Check sheet for the modelled part. Datum: model origin and axes. Units: mm. A direction names the side the tool comes from. Give positions to 0.01 mm unless a question says otherwise; leave off trailing zeros. Loops run counter-clockwise (first coordinate to the right, second up) from the corner with the lowest first, then second, coordinate; pieces in that order, holes last. Notation, with made-up numbers: (58, 26.25) - (114, 26.25) arc R27 ccw to (114, 59.25) - close; hole circle Ø1 at (80, 60). An arc over 180 degrees is marked (long way). Answer in a Markdown table with one row per item. Add a question column.
(1) Thickness scan on L1, parallel to X at y = 1.5, z = 0; L2, parallel to X at y = 4.5, z = 6.25; L3, parallel to Y at x = 3.5, z = -2. Record the ranges inside material, lowest first.
(2) Sectioned sample at D-D on z = -3. Enter the section's corners in (x, y).
(3) Draft check along Z on faces 1 (the face through (8.259, 2.251, -3.307)), 2 (the face through (0.1, 1.8, -6.5)), 3 (the face through (9.5, 4.2, 0.1)), 4 (the face through (-8, 4, 0)). Enter one of: released by +Z, released by -Z, zero draft, split by the parting line, or undercut.
(4) Sectioned sample at A-A on x = 0. Enter the section's corners in (y, z), then the cut area to 3 significant figures.
(5) Go/stop test with flat-tipped pins: P1, Ø5, axis at x = 0, z = 0, coming from the +Y side; P2, Ø3, axis at x = -3, y = 5, coming from the +Z side. Record where each tip stops, or that it passes through.
(6) Sectioned sample at B-B on z = 0. Enter the section's corners in (x, y), then the cut area to 3 significant figures.
(7) Set-up check for faces 5 (the face through (7, 5, 0)), 6 (the face through (8.26, 2.24, 3.3)), 7 (the face through (-2.1, 0, -1.4)): record each of +Z, -Z, +X, -X, +Y, -Y from which the full face is reachable in a straight line by a thin tool's end or side.
(8) Sectioned sample at C-C on y = 4.25. Enter the section's corners in (x, z).
from build123d import *

# Parameters (mm, degrees)
SKETCH1_W               = 19
SKETCH1_H               = 13
SKETCH1_R               = 2.159
BOSS_EXTRUDE1_DEPTH     = 2
BOSS_EXTRUDE2_DEPTH     = 19
CUT_EXTRUDE1_DEPTH      = 18.363755354
CUT_EXTRUDE1_DEPTH_BACK = 18.363755354
SKETCH4_W               = 14
SKETCH4_H               = 5
FILLET1_R               = 0.75
CHAMFER1_SIZE           = 0.5


with BuildPart() as part:
    # Sketch1 → Boss-Extrude1 (new body)
    with BuildSketch(Plane(origin=(0, 0, 0), x_dir=(1, 0, 0), z_dir=(0, 1, 0))):
        Rectangle(SKETCH1_W, SKETCH1_H)
        with Locations(Location((0, 0, 0), (0, 0, 270))):
            Circle(SKETCH1_R, mode=Mode.SUBTRACT)
    extrude(amount=BOSS_EXTRUDE1_DEPTH)

    # Sketch2 → Boss-Extrude2 (add)
    with BuildSketch(Plane(origin=(9.5, 0, 0), x_dir=(0, 0, -1), z_dir=(1, 0, 0))):
        with BuildLine():
            Line((-6.5, 5.2), (-6.5, 2))
            Line((-6.5, 2), (-3.5, 2))
            Line((-3.5, 2), (-3.5, 2.7))
            ThreePointArc((-3.5, 2.7), (-3.119238816, 3.619238816), (-2.2, 4))
            Line((-2.2, 4), (2.2, 4))
            ThreePointArc((2.2, 4), (3.119238816, 3.619238816), (3.5, 2.7))
            Line((3.5, 2.7), (3.5, 2))
            Line((3.5, 2), (6.5, 2))
            Line((6.5, 2), (6.5, 5.2))
            ThreePointArc((6.5, 5.2), (6.119238816, 6.119238816), (5.2, 6.5))
            Line((5.2, 6.5), (-5.2, 6.5))
            ThreePointArc((-5.2, 6.5), (-6.119238816, 6.119238816), (-6.5, 5.2))
        make_face()
    extrude(amount=-BOSS_EXTRUDE2_DEPTH)

    # Sketch4 → Cut-Extrude1 (cut, two sides: drawn at the far end of the back side and taken through both)
    with BuildSketch(Plane.XY.offset(6.5).offset(-CUT_EXTRUDE1_DEPTH_BACK)):
        with Locations((0, 4.5)):
            Rectangle(SKETCH4_W, SKETCH4_H)
    extrude(amount=CUT_EXTRUDE1_DEPTH + CUT_EXTRUDE1_DEPTH_BACK, mode=Mode.SUBTRACT)

    # Fillet1
    # the kernel refuses this fillet: 0.75 mm, written as the material it adds along each edge
    with BuildSketch(Plane(origin=(-7, 2, 3.5), x_dir=(1, 0, 0), z_dir=(0, 0, 1)), Plane(origin=(-7, 2, -6.5), x_dir=(1, 0, 0), z_dir=(0, 0, 1))) as fillet1_piece_1:
        with BuildLine():
            CenterArc((FILLET1_R, FILLET1_R), FILLET1_R, 180, 90)
            Line((0, FILLET1_R), (-FILLET1_R * 0.02, FILLET1_R))
            Line((-FILLET1_R * 0.02, FILLET1_R), (-FILLET1_R * 0.02, -FILLET1_R * 0.02))
            Line((-FILLET1_R * 0.02, -FILLET1_R * 0.02), (FILLET1_R, -FILLET1_R * 0.02))
            Line((FILLET1_R, -FILLET1_R * 0.02), (FILLET1_R, 0))
        make_face()
    extrude(amount=3)
    with BuildSketch(Plane(origin=(-7, 2, 3.5), x_dir=(0, 0, -1), z_dir=(-1, 0, 0)), Plane(origin=(9.5, 2, 3.5), x_dir=(0, 0, -1), z_dir=(-1, 0, 0))) as fillet1_piece_2:
        with BuildLine():
            CenterArc((0.752277442, -0.75), FILLET1_R, 90, 95.21590857)
            Line((0.005383046, -0.818181818), (-0.069306394, -0.825))
            ThreePointArc((-0.069306394, -0.825), (-0.075, -0.7), (-0.075, 0))
            Line((-0.075, 0), (0, 0.075))
            Line((0, 0.075), (0.752277442, 0.075))
            Line((0.752277442, 0.075), (0.752277442, 0))
        make_face()
    extrude(amount=2.5)
    with BuildSketch(Plane(origin=(7, 2, 6.5), x_dir=(0, 1, 0), z_dir=(0, 0, -1)), Plane(origin=(7, 2, -3.5), x_dir=(0, 1, 0), z_dir=(0, 0, -1))) as fillet1_piece_3:
        with BuildLine():
            CenterArc((FILLET1_R, -FILLET1_R), FILLET1_R, 90, 90)
            Line((0, -FILLET1_R), (-FILLET1_R * 0.02, -FILLET1_R))
            Line((-FILLET1_R * 0.02, -FILLET1_R), (-FILLET1_R * 0.02, FILLET1_R * 0.02))
            Line((-FILLET1_R * 0.02, FILLET1_R * 0.02), (FILLET1_R, FILLET1_R * 0.02))
            Line((FILLET1_R, FILLET1_R * 0.02), (FILLET1_R, 0))
        make_face()
    extrude(amount=3)
    with BuildSketch(Plane(origin=(9.5, 2, -3.5), x_dir=(0, 0, 1), z_dir=(-1, 0, 0)), Plane(origin=(-7, 2, -3.5), x_dir=(0, 0, 1), z_dir=(-1, 0, 0))) as fillet1_piece_4:
        with BuildLine():
            CenterArc((0.752277442, 0.75), FILLET1_R, 174.78409143, 95.21590857)
            Line((0.005383046, 0.818181818), (-0.069306394, 0.825))
            ThreePointArc((-0.069306394, 0.825), (-0.075, 0.7), (-0.075, 0))
            Line((-0.075, 0), (0, -0.075))
            Line((0, -0.075), (0.752277442, -0.075))
            Line((0.752277442, -0.075), (0.752277442, 0))
        make_face()
    extrude(amount=2.5)
    with BuildSketch(Plane(origin=(-7, 2, 1.625), x_dir=(1, 0, 0), z_dir=(0, 0, 1))) as fillet1_piece_5a_section:
        with BuildLine():
            CenterArc((FILLET1_R, FILLET1_R), FILLET1_R, 180, 90)
            Line((0, FILLET1_R), (-FILLET1_R * 0.02, FILLET1_R))
            Line((-FILLET1_R * 0.02, FILLET1_R), (-FILLET1_R * 0.02, -FILLET1_R * 0.02))
            Line((-FILLET1_R * 0.02, -FILLET1_R * 0.02), (FILLET1_R, -FILLET1_R * 0.02))
            Line((FILLET1_R, -FILLET1_R * 0.02), (FILLET1_R, 0))
        make_face()
    fillet1_piece_5a = extrude(amount=4.875, mode=Mode.PRIVATE)
    fillet1_piece_5a = split(fillet1_piece_5a, bisect_by=Plane(origin=(-6.830203664, 2.169796336, 3.5), z_dir=(0, 0, -1)), keep=Keep.TOP, mode=Mode.PRIVATE)
    with BuildSketch(Plane(origin=(-4.954501184, 2, 3.5), x_dir=(0, 0, -1), z_dir=(-1, 0, 0))) as fillet1_piece_5b_section:
        with BuildLine():
            CenterArc((0.752277442, -0.75), FILLET1_R, 90, 95.21590857)
            Line((0.005383046, -0.818181818), (-0.069306394, -0.825))
            ThreePointArc((-0.069306394, -0.825), (-0.075, -0.7), (-0.075, 0))
            Line((-0.075, 0), (0, 0.075))
            Line((0, 0.075), (0.752277442, 0.075))
            Line((0.752277442, 0.075), (0.752277442, 0))
        make_face()
    fillet1_piece_5b = extrude(amount=4.545498816, mode=Mode.PRIVATE)
    fillet1_piece_5b = split(fillet1_piece_5b, bisect_by=Plane(origin=(-7, 2.182819777, 3.341220423), z_dir=(1, 0, 0)), keep=Keep.TOP, mode=Mode.PRIVATE)
    fillet1_piece_5 = fillet1_piece_5a & fillet1_piece_5b
    add(fillet1_piece_5)
    with BuildSketch(Plane(origin=(7, 2, 6.5), x_dir=(0, 1, 0), z_dir=(0, 0, -1))) as fillet1_piece_6a_section:
        with BuildLine():
            CenterArc((FILLET1_R, -FILLET1_R), FILLET1_R, 90, 90)
            Line((0, -FILLET1_R), (-FILLET1_R * 0.02, -FILLET1_R))
            Line((-FILLET1_R * 0.02, -FILLET1_R), (-FILLET1_R * 0.02, FILLET1_R * 0.02))
            Line((-FILLET1_R * 0.02, FILLET1_R * 0.02), (FILLET1_R, FILLET1_R * 0.02))
            Line((FILLET1_R, FILLET1_R * 0.02), (FILLET1_R, 0))
        make_face()
    fillet1_piece_6a = extrude(amount=4.875, mode=Mode.PRIVATE)
    fillet1_piece_6a = split(fillet1_piece_6a, bisect_by=Plane(origin=(6.830203664, 2.169796336, 3.5), z_dir=(0, 0, -1)), keep=Keep.TOP, mode=Mode.PRIVATE)
    with BuildSketch(Plane(origin=(9.5, 2, 3.5), x_dir=(0, 0, -1), z_dir=(-1, 0, 0))) as fillet1_piece_6b_section:
        with BuildLine():
            CenterArc((0.752277442, -0.75), FILLET1_R, 90, 95.21590857)
            Line((0.005383046, -0.818181818), (-0.069306394, -0.825))
            ThreePointArc((-0.069306394, -0.825), (-0.075, -0.7), (-0.075, 0))
            Line((-0.075, 0), (0, 0.075))
            Line((0, 0.075), (0.752277442, 0.075))
            Line((0.752277442, 0.075), (0.752277442, 0))
        make_face()
    fillet1_piece_6b = extrude(amount=4.545498816, mode=Mode.PRIVATE)
    fillet1_piece_6b = split(fillet1_piece_6b, bisect_by=Plane(origin=(7, 2.182819777, 3.341220423), z_dir=(-1, 0, 0)), keep=Keep.TOP, mode=Mode.PRIVATE)
    fillet1_piece_6 = fillet1_piece_6a & fillet1_piece_6b
    add(fillet1_piece_6)
    with BuildSketch(Plane(origin=(7, 2, -1.625), x_dir=(0, 1, 0), z_dir=(0, 0, -1))) as fillet1_piece_7a_section:
        with BuildLine():
            CenterArc((FILLET1_R, -FILLET1_R), FILLET1_R, 90, 90)
            Line((0, -FILLET1_R), (-FILLET1_R * 0.02, -FILLET1_R))
            Line((-FILLET1_R * 0.02, -FILLET1_R), (-FILLET1_R * 0.02, FILLET1_R * 0.02))
            Line((-FILLET1_R * 0.02, FILLET1_R * 0.02), (FILLET1_R, FILLET1_R * 0.02))
            Line((FILLET1_R, FILLET1_R * 0.02), (FILLET1_R, 0))
        make_face()
    fillet1_piece_7a = extrude(amount=4.875, mode=Mode.PRIVATE)
    fillet1_piece_7a = split(fillet1_piece_7a, bisect_by=Plane(origin=(6.830203664, 2.169796336, -3.5), z_dir=(0, 0, 1)), keep=Keep.TOP, mode=Mode.PRIVATE)
    with BuildSketch(Plane(origin=(9.5, 2, -3.5), x_dir=(0, 0, 1), z_dir=(-1, 0, 0))) as fillet1_piece_7b_section:
        with BuildLine():
            CenterArc((0.752277442, 0.75), FILLET1_R, 174.78409143, 95.21590857)
            Line((0.005383046, 0.818181818), (-0.069306394, 0.825))
            ThreePointArc((-0.069306394, 0.825), (-0.075, 0.7), (-0.075, 0))
            Line((-0.075, 0), (0, -0.075))
            Line((0, -0.075), (0.752277442, -0.075))
            Line((0.752277442, -0.075), (0.752277442, 0))
        make_face()
    fillet1_piece_7b = extrude(amount=4.545498816, mode=Mode.PRIVATE)
    fillet1_piece_7b = split(fillet1_piece_7b, bisect_by=Plane(origin=(7, 2.182819777, -3.341220423), z_dir=(-1, 0, 0)), keep=Keep.TOP, mode=Mode.PRIVATE)
    fillet1_piece_7 = fillet1_piece_7a & fillet1_piece_7b
    add(fillet1_piece_7)
    with BuildSketch(Plane(origin=(-4.954501184, 2, -3.5), x_dir=(0, 0, 1), z_dir=(-1, 0, 0))) as fillet1_piece_8a_section:
        with BuildLine():
            CenterArc((0.752277442, 0.75), FILLET1_R, 174.78409143, 95.21590857)
            Line((0.005383046, 0.818181818), (-0.069306394, 0.825))
            ThreePointArc((-0.069306394, 0.825), (-0.075, 0.7), (-0.075, 0))
            Line((-0.075, 0), (0, -0.075))
            Line((0, -0.075), (0.752277442, -0.075))
            Line((0.752277442, -0.075), (0.752277442, 0))
        make_face()
    fillet1_piece_8a = extrude(amount=4.545498816, mode=Mode.PRIVATE)
    fillet1_piece_8a = split(fillet1_piece_8a, bisect_by=Plane(origin=(-7, 2.182819777, -3.341220423), z_dir=(1, 0, 0)), keep=Keep.TOP, mode=Mode.PRIVATE)
    with BuildSketch(Plane(origin=(-7, 2, -6.5), x_dir=(1, 0, 0), z_dir=(0, 0, 1))) as fillet1_piece_8b_section:
        with BuildLine():
            CenterArc((FILLET1_R, FILLET1_R), FILLET1_R, 180, 90)
            Line((0, FILLET1_R), (-FILLET1_R * 0.02, FILLET1_R))
            Line((-FILLET1_R * 0.02, FILLET1_R), (-FILLET1_R * 0.02, -FILLET1_R * 0.02))
            Line((-FILLET1_R * 0.02, -FILLET1_R * 0.02), (FILLET1_R, -FILLET1_R * 0.02))
            Line((FILLET1_R, -FILLET1_R * 0.02), (FILLET1_R, 0))
        make_face()
    fillet1_piece_8b = extrude(amount=4.875, mode=Mode.PRIVATE)
    fillet1_piece_8b = split(fillet1_piece_8b, bisect_by=Plane(origin=(-6.830203664, 2.169796336, -3.5), z_dir=(0, 0, 1)), keep=Keep.TOP, mode=Mode.PRIVATE)
    fillet1_piece_8 = fillet1_piece_8a & fillet1_piece_8b
    add(fillet1_piece_8)

    # Chamfer1
    chamfer1_edges = [part.edges().sort_by_distance(p)[0] for p in [
        (0, 0, 6.5),
        (-9.5, 0, 0),
        (0, 0, -6.5),
        (9.5, 0, 0),
    ]]
    chamfer(chamfer1_edges, length=CHAMFER1_SIZE)


solid = part.part
Reply:
| question | item | result |
|---|---|---|
| 1 | L1 | -9.5 to -2.16, 2.16 to 9.5 |
| 1 | L2 | -9.5 to -7, 7 to 9.5 |
| 1 | L3 | 0 to 2 |
| 2 | outline | (-9.5, 0.5) - (-9, 0) - (9, 0) - (9.5, 0.5) - (9.5, 2.04) - (6.5, 2.04) arc R0.75 cw to (6.25, 2) - (-6.25, 2) arc R0.75 cw to (-6.5, 2.04) - (-9.5, 2.04) - close; (-9.5, 3.72) - (-7, 3.72) - (-7, 6.5) - (-9.5, 6.5) - close; (7, 3.72) - (9.5, 3.72) - (9.5, 6.5) - (7, 6.5) - close |
| 3 | face 1 | undercut |
| 3 | face 2 | released by -Z |
| 3 | face 3 | zero draft |
| 3 | face 4 | undercut |
| 4 | outline | (0, -6) - (0.5, -6.5) - (2, -6.5) - (2, -2.16) - (0, -2.16) - close; (0, 2.16) - (2, 2.16) - (2, 6.5) - (0.5, 6.5) - (0, 6) - close |
| 4 | area | 17.1 mm^2 |
| 5 | P1 | y = 2 |
| 5 | P2 | through |
| 6 | outline | (-9.5, 0.5) - (-9, 0) - (-2.16, 0) - (-2.16, 2) - (-9.5, 2) - close; (-9.5, 4) - (-7, 4) - (-7, 6.5) - (-9.5, 6.5) - close; (2.16, 0) - (9, 0) - (9.5, 0.5) - (9.5, 2) - (2.16, 2) - close; (7, 4) - (9.5, 4) - (9.5, 6.5) - (7, 6.5) - close |
| 6 | area | 41.6 mm^2 |
| 7 | face 5 | +Z, -Z, +Y |
| 7 | face 6 | +X, -X |
| 7 | face 7 | +Z, -Z, +X, -X, -Y |
| 8 | outline | (-9.5, -6.5) - (-7, -6.5) - (-7, 6.5) - (-9.5, 6.5) - close; (7, -6.5) - (9.5, -6.5) - (9.5, 6.5) - (7, 6.5) - close |
